from build123d import *

# Parameters (mm, degrees)
F0_W     = 33
F0_H     = 33
F1_DEPTH = 2.5
F0_W_2   = 53
F0_H_2   = 53
F0_W_3   = 49.5
F0_H_3   = 49.5
F2_DEPTH = 9
F3_W     = 4
F3_H     = 0.85
F4_DEPTH = 6.75
F5_DEPTH = 2.5
F6_DEPTH = 1.25


with BuildPart() as f1:
    # F0 (on Front) → F1 (new body)
    with BuildSketch(Plane.XZ):
        with BuildLine():
            Line((-20.5, -20.5), (20.5, -20.5))
            Line((20.5, -20.5), (20.5, -3.5))
            ThreePointArc((20.5, -3.5), (17, 0), (20.5, 3.5))
            Line((20.5, 3.5), (20.5, 20.5))
            Line((20.5, 20.5), (-20.5, 20.5))
            Line((-20.5, 20.5), (-20.5, 3.5))
            ThreePointArc((-20.5, 3.5), (-18.0251262658, 2.4748737342), (-17, 0))
            ThreePointArc((-17, 0), (-18.0251262658, -2.4748737342), (-20.5, -3.5))
            Line((-20.5, -3.5), (-20.5, -20.5))
        make_face()
        Rectangle(F0_W, F0_H, mode=Mode.SUBTRACT)
    extrude(amount=F1_DEPTH)

    # F0 (on Front) → F2 (join)
    with BuildSketch(Plane.XZ):
        Rectangle(F0_W_2, F0_H_2)
        Rectangle(F0_W_3, F0_H_3, mode=Mode.SUBTRACT)
        Rectangle(F0_W_3, F0_H_3)
        with BuildLine():
            Line((20.5, -3.5), (20.5, -20.5))
            Line((20.5, -20.5), (-20.5, -20.5))
            Line((-20.5, -20.5), (-20.5, -3.5))
            ThreePointArc((-20.5, -3.5), (-24, 0), (-20.5, 3.5))
            Line((-20.5, 3.5), (-20.5, 20.5))
            Line((-20.5, 20.5), (20.5, 20.5))
            Line((20.5, 20.5), (20.5, 3.5))
            ThreePointArc((20.5, 3.5), (22.9748737342, 2.4748737342), (24, 0))
            ThreePointArc((24, 0), (22.9748737342, -2.4748737342), (20.5, -3.5))
        make_face(mode=Mode.SUBTRACT)
    extrude(amount=F2_DEPTH)

    # F3 (on face) → F4 (cut)
    with BuildSketch(Plane.XY.offset(26.5)):
        with Locations((0, -8.575)):
            Rectangle(F3_W, F3_H)
    extrude(amount=-F4_DEPTH, mode=Mode.SUBTRACT)

    # F0 (on Front) → F5 (join)
    with BuildSketch(Plane.XZ):
        with BuildLine():
            ThreePointArc((20.5, 3.5), (17, 0), (20.5, -3.5))
            Line((20.5, -3.5), (20.5, -1.875))
            ThreePointArc((20.5, -1.875), (18.625, 0), (20.5, 1.875))
            Line((20.5, 1.875), (20.5, 3.5))
        make_face()
        with BuildLine():
            Line((20.5, -1.875), (20.5, -3.5))
            ThreePointArc((20.5, -3.5), (22.9748737342, -2.4748737342), (24, 0))
            ThreePointArc((24, 0), (22.9748737342, 2.4748737342), (20.5, 3.5))
            Line((20.5, 3.5), (20.5, 1.875))
            ThreePointArc((20.5, 1.875), (21.8258252147, 1.3258252147), (22.375, 0))
            ThreePointArc((22.375, 0), (21.8258252147, -1.3258252147), (20.5, -1.875))
        make_face()
        with BuildLine():
            Line((-20.5, -1.875), (-20.5, -3.5))
            ThreePointArc((-20.5, -3.5), (-18.0251262658, -2.4748737342), (-17, 0))
            ThreePointArc((-17, 0), (-18.0251262658, 2.4748737342), (-20.5, 3.5))
            Line((-20.5, 3.5), (-20.5, 1.875))
            ThreePointArc((-20.5, 1.875), (-19.1741747853, 1.3258252147), (-18.625, 0))
            ThreePointArc((-18.625, 0), (-19.1741747853, -1.3258252147), (-20.5, -1.875))
        make_face()
        with BuildLine():
            ThreePointArc((-20.5, 3.5), (-24, 0), (-20.5, -3.5))
            Line((-20.5, -3.5), (-20.5, -1.875))
            ThreePointArc((-20.5, -1.875), (-22.375, 0), (-20.5, 1.875))
            Line((-20.5, 1.875), (-20.5, 3.5))
        make_face()
    extrude(amount=F5_DEPTH)

    # F0 (on Front) → F6 (cut)
    with BuildSketch(Plane.XZ):
        with BuildLine():
            ThreePointArc((20.5, 3.5), (17, 0), (20.5, -3.5))
            Line((20.5, -3.5), (20.5, -1.875))
            ThreePointArc((20.5, -1.875), (18.625, 0), (20.5, 1.875))
            Line((20.5, 1.875), (20.5, 3.5))
        make_face()
        with BuildLine():
            Line((20.5, -1.875), (20.5, -3.5))
            ThreePointArc((20.5, -3.5), (22.9748737342, -2.4748737342), (24, 0))
            ThreePointArc((24, 0), (22.9748737342, 2.4748737342), (20.5, 3.5))
            Line((20.5, 3.5), (20.5, 1.875))
            ThreePointArc((20.5, 1.875), (21.8258252147, 1.3258252147), (22.375, 0))
            ThreePointArc((22.375, 0), (21.8258252147, -1.3258252147), (20.5, -1.875))
        make_face()
        with BuildLine():
            Line((-20.5, -1.875), (-20.5, -3.5))
            ThreePointArc((-20.5, -3.5), (-18.0251262658, -2.4748737342), (-17, 0))
            ThreePointArc((-17, 0), (-18.0251262658, 2.4748737342), (-20.5, 3.5))
            Line((-20.5, 3.5), (-20.5, 1.875))
            ThreePointArc((-20.5, 1.875), (-19.1741747853, 1.3258252147), (-18.625, 0))
            ThreePointArc((-18.625, 0), (-19.1741747853, -1.3258252147), (-20.5, -1.875))
        make_face()
        with BuildLine():
            ThreePointArc((-20.5, 3.5), (-24, 0), (-20.5, -3.5))
            Line((-20.5, -3.5), (-20.5, -1.875))
            ThreePointArc((-20.5, -1.875), (-22.375, 0), (-20.5, 1.875))
            Line((-20.5, 1.875), (-20.5, 3.5))
        make_face()
    extrude(amount=F6_DEPTH, mode=Mode.SUBTRACT)


solid = f1.part
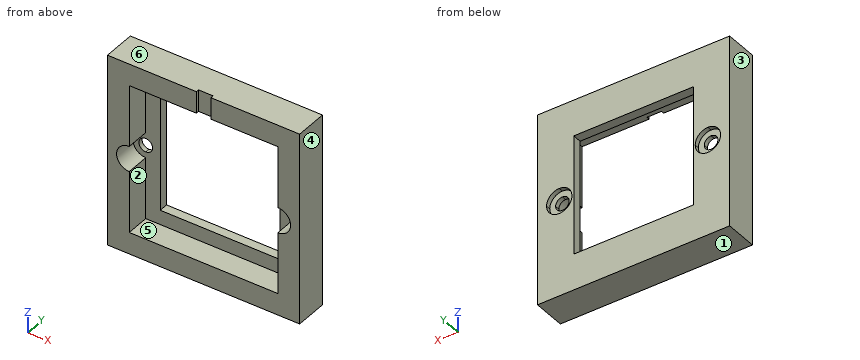
For this review, take the finished solid that the model builds, in its own axes (mm). Face numbers are marked on the shaded views. A direction names the side the tool comes from. Coordinates: 2 decimals unless noted, no trailing zeros. Loops run counter-clockwise (first coordinate to the right, second up) from the corner with the lowest first, then second, coordinate; pieces in that order, holes last. Notation, with made-up numbers: (7.5, -34.5) - (16.5, -34.5) arc R25 ccw to (16.5, -17.5) - close; hole circle Ø7 at (10, -29.5). An arc over 180 degrees is marked (long way). Return JSON: item names as keys, results as strings.
Item 1: Mouldability with a two-part tool opening along X and no side actions: class the marked faces 1, 2, 3 and 4 as pulls with the +X half, pulls with the -X half, needs draft (parallel to the pull), parting line crosses it, or undercut.
Determined:
{"face 1": "needs draft", "face 2": "undercut", "face 3": "pulls with the -X half", "face 4": "pulls with the +X half"}
Item 2: For line 1 (Z direction, x = 15, y = -4.5); line 2 (Z direction, x = 6.5, y = -1.5), list the stretches that pass through material, from the lowest coordinate up.
Determined:
{"line 1": "z = -26.5 to -20.5, 20.5 to 26.5", "line 2": "z = -26.5 to -16.5, 16.5 to 26.5"}
Item 3: For the marked faces 5 and 6, list the 3-axis set-ups (+Z, -Z, +X, -X, +Y, -Y) from which the entire face can be reached by the end or side of a thin tool; tool diameter is ignored.
Determined:
{"face 5": "-Y", "face 6": "+Z, +X, -X, +Y, -Y"}
Item 4: Insertion check: pin 1 (2 mm diameter, centred on x = -0.5, z = 25, fed in from -Y); pin 2 (1.5 mm diameter, centred on x = -3, z = -19.5, fed in from -Y). Each pin has a flat end and moves straight along its axis. Give the tip position at first contact, or say it passes through.
Determined:
{"pin 1": "stops at y = -8.15", "pin 2": "stops at y = -2.5"}
Item 5: Take a section at C-C (y = -5.25). Give the boundary of the cut face in (x, z).
Determined:
{"outline": "(-26.5, -26.5) - (26.5, -26.5) - (26.5, 26.5) - (-26.5, 26.5) - close; hole (-20.5, -20.5) - (20.5, -20.5) - (20.5, -3.5) arc R3.5 ccw to (20.5, 3.5) - (20.5, 20.5) - (-20.5, 20.5) - (-20.5, 3.5) arc R3.5 ccw to (-20.5, -3.5) - close"}
Item 6: Take a section at A-A (z = -12). Give the boundary of the cut face in (x, y), then the cut area to 3 significant figures.
Determined:
{"outline": "(-26.5, -9) - (-20.5, -9) - (-20.5, -2.5) - (-16.5, -2.5) - (-16.5, 0) - (-26.5, 0) - close; (16.5, -2.5) - (20.5, -2.5) - (20.5, -9) - (26.5, -9) - (26.5, 0) - (16.5, 0) - close", "area": "128 mm2"}
Item 7: Take a section at B-B (x = 3). Give the boundary of the cut face in (y, z).
Determined:
{"outline": "(-9, -26.5) - (0, -26.5) - (0, -16.5) - (-2.5, -16.5) - (-2.5, -20.5) - (-9, -20.5) - close; (-9, 20.5) - (-2.5, 20.5) - (-2.5, 16.5) - (0, 16.5) - (0, 26.5) - (-9, 26.5) - close"}
